The listing builds one solid part. Answer for the finished solid, in the listing's coordinates (mm). Face numbers are marked on the shaded views. A direction names the side the tool comes from. Round coordinates to 2 decimals unless told otherwise and drop trailing zeros. Loops run counter-clockwise (first coordinate to the right, second up) from the corner with the lowest first, then second, coordinate; pieces in that order, holes last. Notation, with made-up numbers: M 0.25,-16 L 15.25,-16 A28 cw 15.25,4 Z; hole C 40.25,3 d7. An arc over 180 degrees is marked long. Put each result on its own line as item: value. Start each with the question number.
(1) Section D-D, the plane y = 3 is taken. Determine the outline of the cut face in (x, z), then the cut area to 3 significant figures.
(2) Section A-A, the plane y = 1.35 is taken. Determine the outline of the cut face in (x, z).
(3) Flat-ended cylindrical pins translate along their axes: P1, Ø1.5, axis at y = 0.5, z = 1, coming from the +X side; P2, Ø1.5, axis at x = -4, z = -2, coming from the -Y side. Find the tip coordinate at first contact, or state that the pin passes through.
(4) Section C-C, the plane x = 0 is taken. Determine the outline of the cut face in (y, z), then the cut area to 3 significant figures.
(5) Which of the six approach directions +Z, -Z, +X, -X, +Y, -Y give full straight-line access (tool end or side, diameter ignored) to the marked faces 1, 2, 3, 4 and 5?
(6) Straight lines are drawn through the part: line 1 (Z direction, x = -1.75, y = 1.15); line 2 (Y direction, x = 1.25, z = 3.75). For each, find the intervals that lie inside material, in ascending order.
(7) Section B-B, the plane z = 2.25 is taken. Determine the outline of the cut face in (x, y), then the cut area to 3 significant figures.
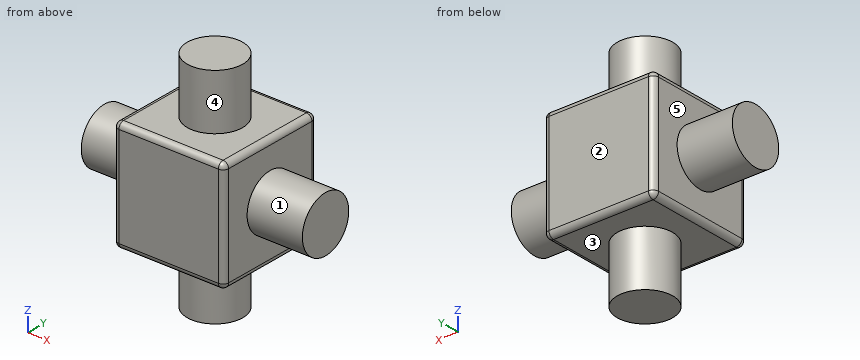
```python
from build123d import *

# Parameters (mm, degrees)
SKETCH1_W           = 6
SKETCH1_H           = 6
BOSS_EXTRUDE1_DEPTH = 6
FILLET1_R           = 0.3
SKETCH2_R           = 1.5
BOSS_EXTRUDE2_DEPTH = 3
CIRPATTERN1_COUNT   = 4


with BuildPart() as part:
    # Sketch1 → Boss-Extrude1 (new body)
    with BuildSketch(Plane(origin=(0, 0, 0), x_dir=(1, 0, 0), z_dir=(0, 1, 0))):
        Rectangle(SKETCH1_W, SKETCH1_H)
    extrude(amount=BOSS_EXTRUDE1_DEPTH)

    # Fillet1
    fillet1_edges = [part.edges().sort_by_distance(p)[0] for p in [
        (-3, 6, 0),
        (0, 6, 3),
        (3, 6, 0),
        (0, 0, 3),
        (-3, 0, 0),
        (0, 0, -3),
        (3, 0, 0),
        (3, 3, 3),
        (-3, 3, 3),
        (-3, 3, -3),
        (3, 3, -3),
        (0, 6, -3),
    ]]
    fillet(fillet1_edges, radius=FILLET1_R)

    # Sketch2 → Boss-Extrude2 (add)
    with BuildSketch(Plane(origin=(0, 0, -3), x_dir=(-1, 0, 0), z_dir=(0, 0, -1))):
        with Locations(Location((0, 3, 0), (0, 0, 180))):
            Circle(SKETCH2_R)
    boss_extrude2 = extrude(amount=BOSS_EXTRUDE2_DEPTH)

    # CirPattern1: Boss-Extrude2 ×4 about axis
    cirpattern1_axis = Axis((0, 0, 0), (0, 1, 0))
    for i in range(1, CIRPATTERN1_COUNT):
        add(boss_extrude2.rotate(cirpattern1_axis, i * 360 / CIRPATTERN1_COUNT))


solid = part.part
```
Recorded:
1. outline: M -6,-1.5 L -3,-1.5 L -3,-2.7 A0.3 ccw -2.7,-3 L -1.5,-3 L -1.5,-6 L 1.5,-6 L 1.5,-3 L 2.7,-3 A0.3 ccw 3,-2.7 L 3,-1.5 L 6,-1.5 L 6,1.5 L 3,1.5 L 3,2.7 A0.3 ccw 2.7,3 L 1.5,3 L 1.5,6 L -1.5,6 L -1.5,3 L -2.7,3 A0.3 ccw -3,2.7 L -3,1.5 L -6,1.5 Z
1. area: 71.9 mm²
2. outline: M -3,-2.7 A0.3 ccw -2.7,-3 L 2.7,-3 A0.3 ccw 3,-2.7 L 3,2.7 A0.3 ccw 2.7,3 L -2.7,3 A0.3 ccw -3,2.7 Z
3. P1: stops at x = 3
3. P2: stops at y = 2.17
4. outline: M 0,-2.7 A0.3 ccw 0.3,-3 L 1.5,-3 L 1.5,-6 L 4.5,-6 L 4.5,-3 L 5.7,-3 A0.3 ccw 6,-2.7 L 6,2.7 A0.3 ccw 5.7,3 L 4.5,3 L 4.5,6 L 1.5,6 L 1.5,3 L 0.3,3 A0.3 ccw 0,2.7 Z
4. area: 53.9 mm²
5. face 1: +X
5. face 2: +Z, -Z, +X, -X, +Y
5. face 3: -Z
5. face 4: +Z
5. face 5: -X
6. line 1: z = -3 to 3
6. line 2: y = 2.17 to 3.83
7. outline: M -3,0.3 A0.3 ccw -2.7,0 L 2.7,0 A0.3 ccw 3,0.3 L 3,5.7 A0.3 ccw 2.7,6 L -2.7,6 A0.3 ccw -3,5.7 Z
7. area: 35.9 mm²
